from build123d import *

# Parameters (mm, degrees)
F1_DEPTH = 107
F2_DEPTH = 17.5
F3_R     = 17.49999


# Not quite as in the source:
# - a fillet or chamfer is up to 0.001 mm smaller than in the source, because OpenCascade refuses the exact size


with BuildPart() as f1:
    # F0 (on Front) → F1 (new body, symmetric)
    with BuildSketch(Plane.XZ):
        with BuildLine():
            ThreePointArc((-109.6174559359, 301.1714849619), (-183.8312478505, -262.5382301946), (320.5, 0))
            ThreePointArc((320.5, 0), (262.5382301946, 183.8312478505), (109.6174559359, 301.1714849619))
            Line((109.6174559359, 301.1714849619), (107.9073522021, 296.4730135685))
            ThreePointArc((107.9073522021, 296.4730135685), (245.7106265432, 197.905362326), (312.6560960166, 42.2659444153))
            ThreePointArc((312.6560960166, 42.2659444153), (312.9876062183, 31.2398034738), (312.3457274768, 20.2273707381))
            ThreePointArc((312.3457274768, 20.2273707381), (312.836389108, 10.1189747444), (313, 0))
            ThreePointArc((313, 0), (-10.1189747444, -312.836389108), (-312.3457274768, 20.2273707381))
            ThreePointArc((-312.3457274768, 20.2273707381), (-312.9876062183, 31.2398034738), (-312.6560960166, 42.2659444153))
            ThreePointArc((-312.6560960166, 42.2659444153), (-245.7106265432, 197.905362326), (-107.9073522021, 296.4730135685))
            Line((-107.9073522021, 296.4730135685), (-109.6174559359, 301.1714849619))
        make_face()
        with BuildLine():
            Line((107.9073522021, 296.4730135685), (109.6174559359, 301.1714849619))
            ThreePointArc((109.6174559359, 301.1714849619), (55.6542409422, 315.6308848404), (0, 320.5))
            Line((0, 320.5), (0, 315.4999911785))
            ThreePointArc((0, 315.4999911785), (54.7859985221, 310.7068373879), (107.9073522021, 296.4730135685))
        make_face()
        with BuildLine():
            Line((-107.0523048609, 294.123790306), (-107.9073522021, 296.4730135685))
            ThreePointArc((-107.9073522021, 296.4730135685), (-245.7106265432, 197.905362326), (-312.6560960166, 42.2659444153))
            ThreePointArc((-312.6560960166, 42.2659444153), (-312.9876062183, 31.2398034738), (-312.3457274768, 20.2273707381))
            ThreePointArc((-312.3457274768, 20.2273707381), (-250.4565621924, 187.7245600735), (-107.0523048609, 294.123790306))
        make_face()
        with BuildLine():
            ThreePointArc((0, 320.5), (-55.6542409423, 315.6308848404), (-109.6174559359, 301.1714849619))
            Line((-109.6174559359, 301.1714849619), (-107.9073522021, 296.4730135685))
            ThreePointArc((-107.9073522021, 296.4730135685), (-54.7859985221, 310.7068373879), (0, 315.4999911785))
            Line((0, 315.4999911785), (0, 320.5))
        make_face()
        with BuildLine():
            ThreePointArc((312.6560960166, 42.2659444153), (245.7106265432, 197.905362326), (107.9073522021, 296.4730135685))
            Line((107.9073522021, 296.4730135685), (107.0523048609, 294.123790306))
            ThreePointArc((107.0523048609, 294.123790306), (250.4565621924, 187.7245600735), (312.3457274768, 20.2273707381))
            ThreePointArc((312.3457274768, 20.2273707381), (312.9876062183, 31.2398034738), (312.6560960166, 42.2659444153))
        make_face()
        with BuildLine():
            ThreePointArc((0, 315.4999911785), (-54.7859985221, 310.7068373879), (-107.9073522021, 296.4730135685))
            Line((-107.9073522021, 296.4730135685), (-107.0523048609, 294.123790306))
            ThreePointArc((-107.0523048609, 294.123790306), (-54.3518796098, 308.2448266928), (0, 313))
            Line((0, 313), (0, 315.4999911785))
        make_face()
        with BuildLine():
            Line((107.0523048609, 294.123790306), (107.9073522021, 296.4730135685))
            ThreePointArc((107.9073522021, 296.4730135685), (54.7859985221, 310.7068373879), (0, 315.4999911785))
            Line((0, 315.4999911785), (0, 313))
            ThreePointArc((0, 313), (54.3518796097, 308.2448266928), (107.0523048609, 294.123790306))
        make_face()
    extrude(amount=F1_DEPTH, both=True)

    # F0 (on Front) → F2 (cut, symmetric)
    with BuildSketch(Plane.XZ):
        with BuildLine():
            ThreePointArc((0, 320.5), (-55.6542409423, 315.6308848404), (-109.6174559359, 301.1714849619))
            Line((-109.6174559359, 301.1714849619), (-107.9073522021, 296.4730135685))
            ThreePointArc((-107.9073522021, 296.4730135685), (-54.7859985221, 310.7068373879), (0, 315.4999911785))
            Line((0, 315.4999911785), (0, 320.5))
        make_face()
        with BuildLine():
            Line((107.9073522021, 296.4730135685), (109.6174559359, 301.1714849619))
            ThreePointArc((109.6174559359, 301.1714849619), (55.6542409422, 315.6308848404), (0, 320.5))
            Line((0, 320.5), (0, 315.4999911785))
            ThreePointArc((0, 315.4999911785), (54.7859985221, 310.7068373879), (107.9073522021, 296.4730135685))
        make_face()
        with BuildLine():
            ThreePointArc((0, 315.4999911785), (-54.7859985221, 310.7068373879), (-107.9073522021, 296.4730135685))
            Line((-107.9073522021, 296.4730135685), (-107.0523048609, 294.123790306))
            ThreePointArc((-107.0523048609, 294.123790306), (-54.3518796098, 308.2448266928), (0, 313))
            Line((0, 313), (0, 315.4999911785))
        make_face()
        with BuildLine():
            Line((107.0523048609, 294.123790306), (107.9073522021, 296.4730135685))
            ThreePointArc((107.9073522021, 296.4730135685), (54.7859985221, 310.7068373879), (0, 315.4999911785))
            Line((0, 315.4999911785), (0, 313))
            ThreePointArc((0, 313), (54.3518796097, 308.2448266928), (107.0523048609, 294.123790306))
        make_face()
        with BuildLine():
            Line((-107.0523048609, 294.123790306), (-107.9073522021, 296.4730135685))
            ThreePointArc((-107.9073522021, 296.4730135685), (-245.7106265432, 197.905362326), (-312.6560960166, 42.2659444153))
            ThreePointArc((-312.6560960166, 42.2659444153), (-312.9876062183, 31.2398034738), (-312.3457274768, 20.2273707381))
            ThreePointArc((-312.3457274768, 20.2273707381), (-250.4565621924, 187.7245600735), (-107.0523048609, 294.123790306))
        make_face()
        with BuildLine():
            ThreePointArc((312.6560960166, 42.2659444153), (245.7106265432, 197.905362326), (107.9073522021, 296.4730135685))
            Line((107.9073522021, 296.4730135685), (107.0523048609, 294.123790306))
            ThreePointArc((107.0523048609, 294.123790306), (250.4565621924, 187.7245600735), (312.3457274768, 20.2273707381))
            ThreePointArc((312.3457274768, 20.2273707381), (312.9876062183, 31.2398034738), (312.6560960166, 42.2659444153))
        make_face()
    extrude(amount=F2_DEPTH, both=True, mode=Mode.SUBTRACT)

    # F3 (radius 17.5 in the source; OpenCascade refuses exactly that, so slightly less here)
    f3_edges = [f1.edges().sort_by_distance(p)[0] for p in [
        (-108.762404, 17.5, 298.822249),
        (108.762404, 17.5, 298.822249),
        (-108.762404, -17.5, 298.822249),
        (108.762404, -17.5, 298.822249),
    ]]
    fillet(f3_edges, radius=F3_R)


solid = f1.part
Can you work these out from the model? Positions are in its coordinate system, mm. A direction names the side the tool comes from. Round coordinates to 2 decimals unless told otherwise and drop trailing zeros. Loops run counter-clockwise (first coordinate to the right, second up) from the corner with the lowest first, then second, coordinate; pieces in that order, holes last. Notation, with made-up numbers: (54.25, 34) - (64.25, 34) arc R17 ccw to (64.25, 60) - close; hole circle Ø11 at (1, 58.5). An arc over 180 degrees is marked (long way). Answer in a Markdown table with one row per item. Add a question column.
Q1. We'd pull the mould along X, two halves only. Please class faces 4 (the flat face through (70, 107, -307)), 5 (the cylindrical face through (-14.09, -1.5, -320.19)), 6 (the flat face through (45, -17.5, 316)): pulls with the +X half, pulls with the -X half, needs draft (parallel to the pull), parting line crosses it, or undercut.
Q2. I want a section at C-C on x = 224.5. List the corners of the cut face in (y, z) for me, and give its area (3 significant figures).
Q3. I need wall thicknesses on L1, parallel to X at y = -26, z = 0; L2, parallel to X at y = -80, z = -278; L3, parallel to Z at x = -98.5, y = 60. Which ranges of each line are inside material? Lowest first, please.
Q4. Which directions (+Z, -Z, +X, -X, +Y, -Y) give clear straight access to the entire face, cutting with the end or side of a thin tool? Please do faces 1 (the cylindrical face through (-103.977, -12.238, 300.265)), 2 (the cylindrical face through (-312.99, -0.25, 31.39)), 3 (the cylindrical face through (13.762, 1.498, -312.697)).
Q5. I want a section at D-D on y = -39.5. List the corners of the cut face in (x, z) for me, and give its area (3 significant figures).
Q6. I want a section at A-A on x = 0. List the corners of the cut face in (y, z) for me, and give its area (3 significant figures).
Q7. I want a section at B-B on z = 0. List the corners of the cut face in (x, y) for me.
Q8. For pin 1 Ø10 at (y, z) = (62, -102.5) entering from -X; pin 2 Ø2 at (y, z) = (61.5, -92.5) entering from +X; pin 3 Ø1 at (y, z) = (57, -72.5) entering from +X, each with a flat end and sliding along its axis, tell me the tip position at first contact or that it passes through.
A:
| question | item | result |
|---|---|---|
| 1 | face 4 | needs draft |
| 1 | face 5 | parting line crosses it |
| 1 | face 6 | undercut |
| 2 | outline | (-107, -228.74) - (107, -228.74) - (107, -218.1) - (-107, -218.1) - close; (-107, 218.1) - (-17.5, 218.1) - (-17.5, 221.68) - (17.5, 221.68) - (17.5, 218.1) - (107, 218.1) - (107, 228.74) - (-107, 228.74) - close |
| 2 | area | 4,430 mm^2 |
| 3 | L1 | -320.5 to -313, 313 to 320.5 |
| 3 | L2 | -159.49 to -143.82, 143.82 to 159.49 |
| 3 | L3 | -304.99 to -297.1, 297.1 to 304.99 |
| 4 | face 1 | +Z |
| 4 | face 2 | none |
| 4 | face 3 | +Y, -Y |
| 5 | outline | circle Ø641 at (0, 0); hole circle Ø626 at (0, 0) |
| 5 | area | 14,900 mm^2 |
| 6 | outline | (-107, -320.5) - (107, -320.5) - (107, -313) - (-107, -313) - close; (-107, 313) - (-17.5, 313) - (-17.5, 320.5) - (-107, 320.5) - close; (17.5, 313) - (107, 313) - (107, 320.5) - (17.5, 320.5) - close |
| 6 | area | 2,950 mm^2 |
| 7 | outline | (-320.5, -107) - (-313, -107) - (-313, 107) - (-320.5, 107) - close; (313, -107) - (320.5, -107) - (320.5, 107) - (313, 107) - close |
| 8 | pin 1 | x = -305.31 |
| 8 | pin 2 | x = 307.16 |
| 8 | pin 3 | x = 312.31 |
